Build history of the part. All positions in model axes, mm. Coordinates: 2 decimals unless noted, no trailing zeros. Order: outer loops, then holes, each group sorted by start corner. A loop starts at its lowest first (then second) coordinate and runs counter-clockwise, first axis right, second up. Notation, with made-up numbers: M 1,3 L 51,3 A24 cw 51,37 Z; hole C 65.5,49.5 d1. An arc over 180 degrees is marked long. Write item = value, one per line. Start each with the question number.
Q1. Drill centre lines: probe 1 along Y at (x, z) = (-77.5, 3.95); probe 2 along X at (y, z) = (18, 3.15); probe 3 along X at (y, z) = (-24, 1.45). Where is each one in solid material? Low to high.
Q2. Pin check, flat tips, straight feed: P1, Ø1.5, axis at x = -98, z = 4, coming from the -Y side; P2, Ø2, axis at y = 14.5, z = 3.5, coming from the +X side; P3, Ø1.5, axis at y = -24, z = 4.5, coming from the -X side. Stop position of each tip, or through.
Q3. Band-saw the part on A-A on y = 20.5. Write the cut outline in (x, z).
Q4. Band-saw the part on D-D on z = 4.1. Write the cut outline in (x, y).
Q5. Band-saw the part on C-C on x = -106. Write the cut outline in (y, z), plus the area to 3 significant figures.
Q6. Band-saw the part on B-B on x = -84.5. Write the cut outline in (y, z).
Q7. Pull direction X, two halves, no side cores. Call faces 1 (the face through (-115.44, -32.12, 2.96)), 2 (the face through (-93.15, -5.71, 2.96)), 3 (the face through (-46.786, -32.764, 2.958)), 4 (the face through (-92, -14, 6)): released by +X, released by -X, zero draft, split by the parting line, or undercut.
```python
from build123d import *

# Parameters (mm, degrees)
F0_R     = 4.6
F0_R_2   = 10.95
F1_DEPTH = 6


with BuildPart() as f1:
    # F0 (on Top) → F1 (new body)
    with BuildSketch(Plane.XY):
        with BuildLine():
            ThreePointArc((-54.33825, -17.126217), (-69.16794, -6.186809), (-73.096568, 11.817531))
            ThreePointArc((-73.096568, 11.817531), (-80.439934, 28.01532), (-89.348044, 12.622498))
            ThreePointArc((-89.348044, 12.622498), (-93.298938, -5.940555), (-108.607333, -17.158822))
            ThreePointArc((-108.607333, -17.158822), (-115.297331, -32.349517), (-98.700652, -32.601591))
            ThreePointArc((-98.700652, -32.601591), (-81.408097, -25.671054), (-63.831793, -31.846683))
            ThreePointArc((-63.831793, -31.846683), (-46.625, -32.522185), (-54.33825, -17.126217))
        make_face()
        with Locations((-106.915409, -26.972435)):
            Circle(F0_R, mode=Mode.SUBTRACT)
        with Locations((-55.028885, -27.102339)):
            Circle(F0_R, mode=Mode.SUBTRACT)
        with Locations((-80.934647, -11.972435)):
            Circle(F0_R_2, mode=Mode.SUBTRACT)
        with Locations((-80.934647, 18.027565)):
            Circle(F0_R, mode=Mode.SUBTRACT)
    extrude(amount=F1_DEPTH)


solid = f1.part
```
Recorded:
q1.probe_1 = -25.88 to -22.37, -1.58 to 14.97, 21.09 to 27.42
q1.probe_2 = -90.93 to -85.53, -76.33 to -70.93
q1.probe_3 = -116.42 to -110.43, -103.4 to -58.43, -51.63 to -45.52
q2.P1 = -32.67
q2.P2 = -71.26
q2.P3 = -116.62
q3.outline = M -90.62,0 L -84.81,0 L -84.81,6 L -90.62,6 Z; M -77.06,0 L -71.25,0 L -71.25,6 L -77.06,6 Z
q4.outline = M -108.61,-17.16 A9.96 ccw long -98.7,-32.6 A26.47 cw -63.83,-31.85 A10 ccw long -54.34,-17.13 A26.14 cw -73.1,11.82 A10 ccw long -89.35,12.62 A26.63 cw Z; hole C -106.92,-26.97 d9.2; hole C -80.93,-11.97 d21.9; hole C -80.93,18.03 d9.2; hole C -55.03,-27.1 d9.2
q5.outline = M -36.89,0 L -31.48,0 L -31.48,6 L -36.89,6 Z; M -22.46,0 L -16.3,0 L -16.3,6 L -22.46,6 Z
q5.area = 69.5 mm2
q6.outline = M -25.92,0 L -22.33,0 L -22.33,6 L -25.92,6 Z; M -1.62,0 L 15.12,0 L 15.12,6 L -1.62,6 Z; M 20.93,0 L 27.37,0 L 27.37,6 L 20.93,6 Z
q7.face_1 = undercut
q7.face_2 = released by -X
q7.face_3 = undercut
q7.face_4 = zero draft
